Autodesk Inventor part; units mm, degrees
ref_plane "YZ Plane" through (0, 0, 0) normal (1, 0, 0) x (0, 1, 0)
ref_plane "XZ Plane" through (0, 0, 0) normal (0, 1, 0) x (-1, 0, 0)
ref_plane "XY Plane" through (0, 0, 0) normal (0, 0, 1) x (1, 0, 0)
sketch "Sketch1" plane through (0, 0, 0) normal (0, 0, 1) x (1, 0, 0)
  line L0 (-34.75, 0) -> (34.75, 0)
  line L1 (-34.75, 0) -> (-34.75, 4)
  line L2 (-34.75, 4) -> (-30.25, 4)
  line L3 (34.75, 0) -> (34.75, 4)
  line L4 (34.75, 4) -> (30.25, 4)
  line L5 (-29, 3) -> (29, 3)
  line L6 (-30.25, 4) -> (-29, 3)
  line L7 (30.25, 4) -> (29, 3)
  point P0 (0, 0)
  dimension "d0" = 69.5
  dimension "d1" = 0
  dimension "d2" = 34.75
  dimension "d3" = 4
  dimension "d4" = 4.5
  dimension "d5" = 4
  dimension "d6" = 4.5
  dimension "d7" = 58
  dimension "d8" = 3
  dimension "d9" = 29
revolve "Revolution1" add sketch "Sketch1" angle 360 about axis through (-34.75, 0, 0) along (1, 0, 0)
sketch "Sketch2" plane through (34.75, 0, 0) normal (1, 0, 0) x (0, 0, -1)
  circle A0 centre (0, 0) radius 1.5
  dimension "d11" = 3
extrude "Extrusion1" cut sketch "Sketch2" against normal blind 8
thread "Thread1"
sketch "Sketch3" plane through (-34.75, 0, 0) normal (-1, 0, 0) x (0, 0, 1)
  circle A0 centre (0, 0) radius 1.5
  dimension "d16" = 3
extrude "Extrusion2" cut sketch "Sketch3" against normal blind 8
thread "Thread2"
properties part number "RCT-H010_Al_side_plate_post"
Here's how the part is built. I have some questions about the finished solid (model axes, mm). A direction names the side the tool comes from. Round coordinates to 2 decimals unless told otherwise and drop trailing zeros. Write each loop counter-clockwise with the first axis right and the second up, starting at its lowest first coordinate (ties: lowest second). Pieces come first, ordered by that corner, then holes. Notation, with made-up numbers: (22.25, 38.5) -> (39.25, 38.5) arc R16 ccw to (39.25, 66.5) -> close; hole circle Ø4 at (7, -3). An arc over 180 degrees is marked (long way). One line per item, written item: value.
1) I'm going to push flat-ended pins straight in: pin 1 Ø1.5 at (x, z) = (14.5, -0.5) entering from +Y; pin 2 Ø4 at (x, z) = (7, 1) entering from -Y; pin 3 Ø2.5 at (y, z) = (0, 0) entering from +X. Where does each tip first touch, or does it pass through?
Filled sheet:
pin 1: stops at y = 3
pin 2: stops at y = -3
pin 3: stops at x = 26.75
2) If I drill on line 1 (Z direction, x = -12, y = 0.25); line 2 (X direction, y = -3, z = 2.25); line 3 (X direction, y = -0.5, z = -3), over which ranges is the centre line in solid material (lowest first)? Write a range as [from, to].
Filled sheet:
line 1: z = [-2.99, 2.99]
line 2: x = [-34.75, -29.94], [29.94, 34.75]
line 3: x = [-34.75, -29.05], [29.05, 34.75]
3) Suppose I cut it at A-A on y = 0. List the corners of the cut face in (x, z) for me.
Filled sheet:
outline: (-34.75, -4) -> (-30.25, -4) -> (-29, -3) -> (29, -3) -> (30.25, -4) -> (34.75, -4) -> (34.75, -1.5) -> (26.75, -1.5) -> (26.75, 1.5) -> (34.75, 1.5) -> (34.75, 4) -> (30.25, 4) -> (29, 3) -> (-29, 3) -> (-30.25, 4) -> (-34.75, 4) -> (-34.75, 1.5) -> (-26.75, 1.5) -> (-26.75, -1.5) -> (-34.75, -1.5) -> close
4) For faces 4 (the face through (32.468, -0.867, 3.905)), 5 (the face through (-26.75, 0, 0)), 6 (the face through (30.81, 0.07, 1.5)), which set-ups out of +Z, -Z, +X, -X, +Y, -Y let a thin tool reach every point of the face, with its end or its side?
Filled sheet:
face 4: +X, -X
face 5: -X
face 6: +X
5) We'd pull the mould along Z, two halves only. Please class faces 1 (the face through (0, -3, 0)), 2 (the face through (26.75, 0, 0)), 3 (the face through (-34.75, 2, 0)): released by +Z, released by -Z, zero draft, split by the parting line, or undercut.
Filled sheet:
face 1: split by the parting line
face 2: undercut
face 3: zero draft
6) Suppose I cut it at C-C on x = 24.5. List the corners of the cut face in (y, z) for me.
Filled sheet:
outline: circle Ø6 at (0, 0)
